Geometry check sheet. Reference: the model listing, model coordinates, mm. Face numbers are marked on the shaded views. A direction names the side the tool comes from. Coordinates: 2 decimals unless noted, no trailing zeros. Write each loop counter-clockwise with the first axis right and the second up, starting at its lowest first coordinate (ties: lowest second). Pieces come first, ordered by that corner, then holes. Notation, with made-up numbers: M 69.25,87 L 87.25,87 A30 cw 87.25,110 Z; hole C -2.5,21 d10. An arc over 180 degrees is marked long. Write each question's results on one line, items separated by ' | '.
```python
from build123d import *

# Parameters (mm, degrees)
CYLINDER_R      = 24.765
CYLINDER_DEPTH  = 19.05
SKETCH_R        = 3.175
POCKET_DEPTH    = 19.05
SKETCH001_R     = 25.4
SKETCH001_W     = 9.525
SKETCH001_H     = 9.525
POCKET001_DEPTH = 6.35
SKETCH002_R     = 1.95
HOLE_DEPTH      = 6.810375
HOLE_TIPS_R     = 1.95
CHAMFER_SIZE    = 0.254
FILLET_R        = 0.254
CHAMFER001_SIZE = 0.254


with BuildPart() as part:
    # Cylinder → Cylinder (join)
    with BuildSketch(Plane.XY):
        Circle(CYLINDER_R)
    extrude(amount=CYLINDER_DEPTH)

    # Sketch (on Face3 of Cylinder) → Pocket (cut)
    with BuildSketch(Plane.XY.offset(19.05)):
        with Locations((11.22532, 11.22532)):
            Circle(SKETCH_R)
        with Locations((-11.22532, 11.22532)):
            Circle(SKETCH_R)
        with Locations((-11.22532, -11.22532)):
            Circle(SKETCH_R)
        with Locations((11.22532, -11.22532)):
            Circle(SKETCH_R)
    extrude(amount=-POCKET_DEPTH, mode=Mode.SUBTRACT)

    # Sketch001 (on Face3 of Pocket) → Pocket001 (cut)
    with BuildSketch(Plane.XY.offset(19.05)):
        Circle(SKETCH001_R)
        Rectangle(SKETCH001_W, SKETCH001_H, mode=Mode.SUBTRACT)
        with Locations((0, 16.51)):
            Rectangle(SKETCH001_W, SKETCH001_H, mode=Mode.SUBTRACT)
        with Locations((-16.51, 0)):
            Rectangle(SKETCH001_W, SKETCH001_H, mode=Mode.SUBTRACT)
        with Locations((0, -16.51)):
            Rectangle(SKETCH001_W, SKETCH001_H, mode=Mode.SUBTRACT)
        with Locations((16.51, 0)):
            Rectangle(SKETCH001_W, SKETCH001_H, mode=Mode.SUBTRACT)
    extrude(amount=-POCKET001_DEPTH, mode=Mode.SUBTRACT)

    # Sketch002 (on Face30 of Pocket001) → Hole (cut)
    with BuildSketch(Plane.XY.offset(19.05)):
        with Locations((0, 16.51)):
            Circle(SKETCH002_R)
        with Locations((16.51, 0)):
            Circle(SKETCH002_R)
        with Locations((-16.51, 0)):
            Circle(SKETCH002_R)
        with Locations((0, -16.51)):
            Circle(SKETCH002_R)
        Circle(SKETCH002_R)
    extrude(amount=-HOLE_DEPTH, mode=Mode.SUBTRACT)

    # Hole tips → Hole tip 1 section 0
    with BuildSketch(Plane.XY.offset(12.239625), mode=Mode.PRIVATE) as hole_tip_1_s0:
        with Locations((0, 16.51)):
            Circle(HOLE_TIPS_R)
    loft([hole_tip_1_s0.sketch, Vertex(0, 16.51, 11.067947)], mode=Mode.SUBTRACT)

    # Hole tips → Hole tip 2 section 0
    with BuildSketch(Plane.XY.offset(12.239625), mode=Mode.PRIVATE) as hole_tip_2_s0:
        with Locations((16.51, 0)):
            Circle(HOLE_TIPS_R)
    loft([hole_tip_2_s0.sketch, Vertex(16.51, 0, 11.067947)], mode=Mode.SUBTRACT)

    # Hole tips → Hole tip 3 section 0
    with BuildSketch(Plane.XY.offset(12.239625), mode=Mode.PRIVATE) as hole_tip_3_s0:
        with Locations((-16.51, 0)):
            Circle(HOLE_TIPS_R)
    loft([hole_tip_3_s0.sketch, Vertex(-16.51, 0, 11.067947)], mode=Mode.SUBTRACT)

    # Hole tips → Hole tip 4 section 0
    with BuildSketch(Plane.XY.offset(12.239625), mode=Mode.PRIVATE) as hole_tip_4_s0:
        with Locations((0, -16.51)):
            Circle(HOLE_TIPS_R)
    loft([hole_tip_4_s0.sketch, Vertex(0, -16.51, 11.067947)], mode=Mode.SUBTRACT)

    # Hole tips → Hole tip 5 section 0
    with BuildSketch(Plane.XY.offset(12.239625), mode=Mode.PRIVATE) as hole_tip_5_s0:
        Circle(HOLE_TIPS_R)
    loft([hole_tip_5_s0.sketch, Vertex(0, 0, 11.067947)], mode=Mode.SUBTRACT)

    # Chamfer
    chamfer_edges = [part.edges().sort_by_distance(p)[0] for p in [
        (0, -21.2725, 19.05),
        (-16.51, -4.7625, 19.05),
        (-24.765, 0, 12.7),
        (0, -4.7625, 19.05),
        (0, 11.7475, 19.05),
        (16.51, -4.7625, 19.05),
        (8.05032, 11.22532, 12.7),
        (-14.40032, 11.22532, 12.7),
        (-14.40032, -11.22532, 12.7),
        (8.05032, -11.22532, 12.7),
        (4.7625, -16.51, 19.05),
        (0, -11.7475, 19.05),
        (-4.7625, -16.51, 19.05),
        (-4.7625, 0, 19.05),
        (0, 4.7625, 19.05),
        (4.7625, 0, 19.05),
        (21.2725, 0, 19.05),
        (11.7475, 0, 19.05),
        (16.51, 4.7625, 19.05),
        (-4.7625, 16.51, 19.05),
        (0, 21.2725, 19.05),
        (4.7625, 16.51, 19.05),
        (-11.7475, 0, 19.05),
        (-16.51, 4.7625, 19.05),
        (-21.2725, 0, 19.05),
    ]]
    chamfer(chamfer_edges, length=CHAMFER_SIZE)

    # Fillet
    fillet_edges = [part.edges().sort_by_distance(p)[0] for p in [
        (4.7625, -21.2725, 15.748),
        (4.7625, -11.7475, 15.748),
        (-4.7625, -21.2725, 15.748),
        (-4.7625, -11.7475, 15.748),
        (-21.2725, -4.7625, 15.748),
        (-11.7475, -4.7625, 15.748),
        (-4.7625, -4.7625, 15.748),
        (4.7625, -4.7625, 15.748),
        (11.7475, -4.7625, 15.748),
        (21.2725, -4.7625, 15.748),
        (-4.7625, 11.7475, 15.748),
        (4.7625, 11.7475, 15.748),
        (21.2725, 4.7625, 15.748),
        (11.7475, 4.7625, 15.748),
        (4.7625, 4.7625, 15.748),
        (-4.7625, 4.7625, 15.748),
        (-11.7475, 4.7625, 15.748),
        (-21.2725, 4.7625, 15.748),
        (4.7625, 21.2725, 15.748),
        (-4.7625, 21.2725, 15.748),
    ]]
    fillet(fillet_edges, radius=FILLET_R)

    # Chamfer001
    chamfer001_edges = [part.edges().sort_by_distance(p)[0] for p in [
        (-24.765, 0, 0),
        (8.05032, -11.22532, 0),
        (8.05032, 11.22532, 0),
        (-14.40032, 11.22532, 0),
        (-14.40032, -11.22532, 0),
    ]]
    chamfer(chamfer001_edges, length=CHAMFER001_SIZE)


solid = part.part
```
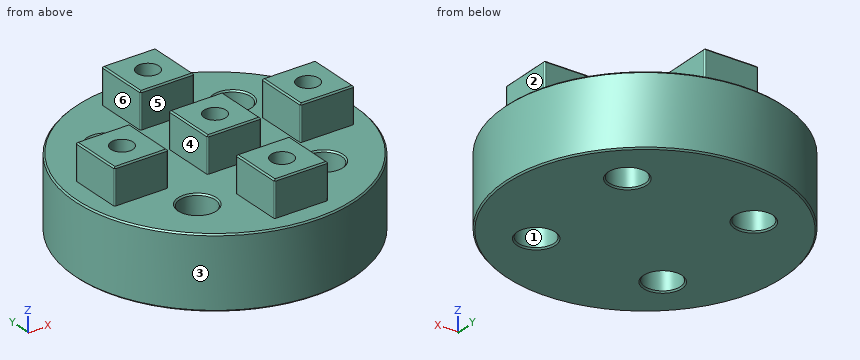
Q1. Access from +Z, -Z, +X, -X, +Y, -Y to the whole of each face (thin tool, end or side, straight path). Record for the marked faces 4, 5 and 6.
Geometry check:
face 4: +Z, +Y, -Y | face 5: +Z, +X, -X | face 6: +Z, -X, +Y, -Y
Q2. Scan lines: probe 1 along Y at (x, z) = (0, 15); probe 2 along X at (y, z) = (2.5, 16.5). Record each from-to range of solid material in increasing order.
Geometry check:
probe 1: y = -21.27 to -18.46, -14.56 to -11.75, -4.76 to -1.95, 1.95 to 4.76, 11.75 to 14.56, 18.46 to 21.27 | probe 2: x = -21.27 to -11.75, -4.76 to 4.76, 11.75 to 21.27
Q3. Mould release check, pull along X, two halves, no side actions. Record for the marked faces 1, 2 and 3: pulls with the +X half, pulls with the -X half, needs draft (parallel to the pull), parting line crosses it, or undercut.
Geometry check:
face 1: undercut | face 2: pulls with the +X half | face 3: parting line crosses it
Q4. Sectioned sample at A-A on z = 16. Give the number of separate pieces and of enclosed holes in the cut face, and give its area (3 significant figures).
Geometry check:
separate pieces: 5 | enclosed holes: 5 | area: 394 mm2
Q5. Sectioned sample at B-B on z = 7.5. Record the cut outline in (x, y) (3 decimals), and give its area (3 significant figures).
Geometry check:
outline: C 0,0 d49.53; hole C -11.225,-11.225 d6.35; hole C -11.225,11.225 d6.35; hole C 11.225,-11.225 d6.35; hole C 11.225,11.225 d6.35 | area: 1,800 mm2
Q6. Depth check by flat-ended pin: P1, Ø3, axis at y = -12.5, z = 7, coming from the -X side; P2, Ø1.8, axis at y = 0, z = 15, coming from the -X side; P3, Ø3, axis at x = 1, z = 17, coming from the -Y side. Enter the tip coordinate at first touch or a pass-through.
Geometry check:
P1: stops at x = -22.19 | P2: stops at x = -21.27 | P3: stops at y = -21.27
